```python
from build123d import *

# Parameters (mm, degrees)
SKETCH1_R                       = 44.45
SKETCH1_R_2                     = 38.1
BOSS_EXTRUDE1_DEPTH             = 203.2
SKETCH2_W                       = 7.89975339
SKETCH2_H                       = 28.462346772
CUT_EXTRUDE1_DEPTH              = 38.1
F_10_32_TAPPED_HOLE1_AT_2_COUNT = 2
F_10_32_TAPPED_HOLE1_AT_2_PITCH = 12.7
F_8_32_TAPPED_HOLE1_D           = 3.4544
F_8_32_TAPPED_HOLE1_DEPTH       = 14.986
F_8_32_TAPPED_HOLE1_TIP         = 1.037806461


with BuildPart() as part:
    # Sketch1 → Boss-Extrude1 (new, symmetric)
    with BuildSketch(Plane.XY):
        Circle(SKETCH1_R)
        Circle(SKETCH1_R_2, mode=Mode.SUBTRACT)
    extrude(amount=BOSS_EXTRUDE1_DEPTH, both=True)

    # Sketch2 → Cut-Extrude1 (cut)
    with BuildSketch(Plane.XY.offset(203.2)):
        with Locations((47.129876695, -0.406604954)):
            Rectangle(SKETCH2_W, SKETCH2_H)
    cut_extrude1 = extrude(amount=-CUT_EXTRUDE1_DEPTH, mode=Mode.SUBTRACT)

    # Sketch3 → #10-32 Tapped Hole1 (revolve, cut)
    with BuildSketch(Plane(origin=(43.18, 0, 193.675), x_dir=(0, 0, -1), z_dir=(0, 1, 0))):
        Polygon((0, 0), (0, 14.929317848), (2.0193, 13.716), (2.0193, 0), align=None)
    f_10_32_tapped_hole1 = revolve(axis=Axis((49.53, 0, 193.675), (-1, 0, 0)), mode=Mode.SUBTRACT)

    # #10-32 Tapped Hole1 at 2: #10-32 Tapped Hole1 ×2
    with Locations(*[(0, 0, -i * F_10_32_TAPPED_HOLE1_AT_2_PITCH) for i in range(1, F_10_32_TAPPED_HOLE1_AT_2_COUNT)]):
        add(f_10_32_tapped_hole1, mode=Mode.SUBTRACT)

    # #8-32 Tapped Hole1
    with Locations(Plane(origin=(0, 0, -203.2), x_dir=(-1, 0, 0), z_dir=(0, 0, -1))):
        with Locations((0, 41.275), (-41.275, 0), (41.275, 0), (0, -41.275)):
            Hole(F_8_32_TAPPED_HOLE1_D / 2, depth=F_8_32_TAPPED_HOLE1_DEPTH)
            with Locations((0, 0, -(F_8_32_TAPPED_HOLE1_DEPTH + F_8_32_TAPPED_HOLE1_TIP / 2))):  # 118° drill point
                Cone(0, F_8_32_TAPPED_HOLE1_D / 2, F_8_32_TAPPED_HOLE1_TIP, mode=Mode.SUBTRACT)

    # Mirror1: Cut-Extrude1, #10-32 Tapped Hole1 across plane
    add(cut_extrude1.mirror(Plane(origin=(0, 0, 0), x_dir=(0, 0, 1), z_dir=(1, 0, 0))), mode=Mode.SUBTRACT)
    add(f_10_32_tapped_hole1.mirror(Plane(origin=(0, 0, 0), x_dir=(0, 0, 1), z_dir=(1, 0, 0))), mode=Mode.SUBTRACT)

    # Mirror1 copy 1 sketch → Mirror1 copy 1 (revolve, cut)
    with BuildSketch(Plane(origin=(-43.18, 0, 180.975), x_dir=(0, 0, -1), z_dir=(0, 1, 0))):
        Polygon((0, 0), (0, -14.929317848), (2.0193, -13.716), (2.0193, 0), align=None)
    revolve(axis=Axis((-49.53, 0, 180.975), (-1, 0, 0)), mode=Mode.SUBTRACT)


solid = part.part
```
Source: CAD feature listing. Evaluate the final solid. Frame: model axes, mm. A direction names the side the tool comes from. Coordinates: 2 decimals unless noted, no trailing zeros. Loops run counter-clockwise (first coordinate to the right, second up) from the corner with the lowest first, then second, coordinate; pieces in that order, holes last. Notation, with made-up numbers: (20, 73) -> (76, 73) arc R22 ccw to (76, 96) -> close; hole circle Ø4 at (74.5, -29). An arc over 180 degrees is marked (long way). One line per item, written item: value. Start each with the question number.
Q1. Line query: line 1 along Y through (x, z) = (0, 96); line 2 along X through (y, z) = (2.5, 176); line 3 along X through (y, z) = (-13.5, -42). Output: solid intervals per line, ascending.
Q2. Section query A-A, the plane x = -31. Return the cut outline in (y, z), and give its area (3 significant figures).
Q3. Section query C-C, the plane y = 23.5. Return the cut outline in (x, z), and give its area (3 significant figures).
Q4. Section query B-B, the plane z = -59. Return the cut outline in (x, y), and give its area (3 significant figures).
Q5. Set-up query: faces 4 (the face through (-43.18, 0, 184)), 5 (the face through (13, 36, 203.2)), 6 (the face through (43.18, 0, 184)). Return all of +Z, -Z, +X, -X, +Y, -Y with unobstructed straight access to the full face (end or side cutting, diameter ignored); none if empty.
Q6. Mould query, pull axis Y, two halves, no side actions, for faces 1 (the face through (42.397, 13.352, 2.845)), 2 (the face through (-30.235, -23.183, -2.845)), 3 (the face through (20, -33, -203.2)). Classes: pulls with the +Y half, pulls with the -Y half, needs draft (parallel to the pull), parting line crosses it, or undercut.
Q7. Contact query for flat-ended pins moving along their axis: P1, Ø1, axis at x = -18.5, z = 102, coming from the +Y side; P2, Ø4, axis at x = -21, z = 147.5, coming from the +Y side; P3, Ø0.6, axis at x = 44, y = -4.5, coming from the +Z side; P4, Ø8, axis at y = -1, z = 82.5, coming from the -X side. Output: stop coordinate, or through.
Results:
1. line 1: -44.45 to -38.1, 38.1 to 44.45
1. line 2: -43.18 to -38.02, 38.02 to 43.18
1. line 3: -42.35 to -35.63, 35.63 to 42.35
2. outline: (-31.86, -203.2) -> (-22.15, -203.2) -> (-22.15, 203.2) -> (-31.86, 203.2) -> close; (22.15, -203.2) -> (31.86, -203.2) -> (31.86, 203.2) -> (22.15, 203.2) -> close
2. area: 7,890 mm^2
3. outline: (-37.73, -203.2) -> (-29.99, -203.2) -> (-29.99, 203.2) -> (-37.73, 203.2) -> close; (29.99, -203.2) -> (37.73, -203.2) -> (37.73, 203.2) -> (29.99, 203.2) -> close
3. area: 6,290 mm^2
4. outline: circle Ø88.9 at (0, 0); hole circle Ø76.2 at (0, 0)
4. area: 1,650 mm^2
5. face 4: +Z, -X, +Y, -Y
5. face 5: +Z, +X, -X, +Y, -Y
5. face 6: +Z, +X, +Y, -Y
6. face 1: parting line crosses it
6. face 2: undercut
6. face 3: needs draft
7. P1: y = 40.64
7. P2: y = 40.18
7. P3: z = 165.1
7. P4: x = -44.45
